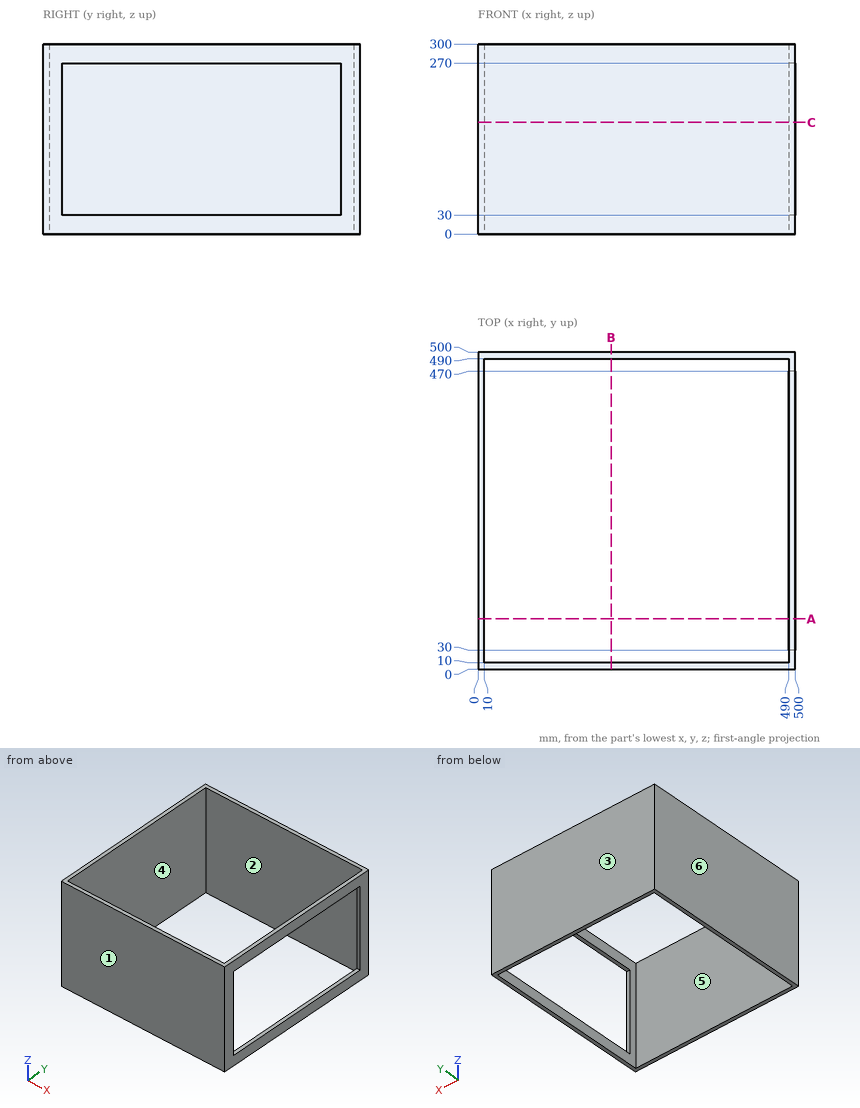
Study the drawing (mm; zero at the part's minimum x, y, z) and answer. A direction names the side the tool comes from. Round coordinates to 2 decimals unless told otherwise and drop trailing zeros. Loops run counter-clockwise (first coordinate to the right, second up) from the corner with the lowest first, then second, coordinate; pieces in that order, holes last. Notation, with made-up numbers: (28.25, 57.5) -> (38.25, 57.5) arc R25 cw to (38.25, 83.5) -> close; hole circle Ø6 at (26, 4). An arc over 180 degrees is marked (long way). Write each question's results on one line, items separated by ' | '. Start each with the question number.
1. A tool of negligible diameter and unlimited length cuts with its end or side. For the marked faces 1 and 2, from which of +Z, -Z, +X, -X, +Y, -Y can it reach the whole face along a straight path? Write none if from no direction.
2. For a pull along Y with two mould halves and no side action, classify the marked faces 3, 4, 5 and 6 as +Y half, -Y half, draft (parallel to the pull), parting line (faces both ways), or undercut.
3. Section C-C (z = 176.5) is taken. Determine the outline of the cut face in (x, y).
4. Section B-B (x = 210) is taken. Determine the outline of the cut face in (y, z).
5. Find the intervals of material crossed by probe 1 along Y at (x, z) = (453, 32); probe 2 along X at (y, z) = (402.5, 229), in increasing order. Write a range as from..to.
6. Given pin 1 Ø2 at (y, z) = (55.5, 117) entering from +X, flat-ended and moving along its own axis, determine where the tip first touches the part or whether it passes through.
7. Section A-A (y = 79.5) is taken. Determine the outline of the cut face in (x, z).
Evaluation:
1) face 1: +Z, -Z, +X, -X, -Y | face 2: +Z, -Z
2) face 3: +Y half | face 4: undercut | face 5: undercut | face 6: draft
3) outline: (0, 0) -> (500, 0) -> (500, 30) -> (490, 30) -> (490, 10) -> (10, 10) -> (10, 490) -> (490, 490) -> (490, 470) -> (500, 470) -> (500, 500) -> (0, 500) -> close
4) outline: (0, 0) -> (10, 0) -> (10, 300) -> (0, 300) -> close; (490, 0) -> (500, 0) -> (500, 300) -> (490, 300) -> close
5) probe 1: y = 0..10, 490..500 | probe 2: x = 0..10
6) pin 1: stops at x = 10
7) outline: (0, 0) -> (10, 0) -> (10, 300) -> (0, 300) -> close; (490, 0) -> (500, 0) -> (500, 30) -> (490, 30) -> close; (490, 270) -> (500, 270) -> (500, 300) -> (490, 300) -> close
